from build123d import *

# Parameters (mm, degrees)
SKETCH_W     = 250
SKETCH_H     = 10
SKETCH001_R  = 60
PAD_DEPTH    = 60
SKETCH002_R  = 45
PAD001_DEPTH = 45
SKETCH003_R  = 45
PAD002_DEPTH = 20


with BuildPart() as part:
    # Sketch → Revolution (revolve)
    with BuildSketch(Plane.XY):
        with Locations((125, 35)):
            Rectangle(SKETCH_W, SKETCH_H)
    revolve(axis=Axis((0, 0, 0), (1, 0, 0)))

    # Sketch001 → Pad (new body, symmetric)
    with BuildSketch(Plane.XY):
        Circle(SKETCH001_R)
    extrude(amount=PAD_DEPTH, both=True)

    # Sketch002 → Pad001 (join, symmetric)
    with BuildSketch(Plane.XY):
        with Locations((250, 0)):
            Circle(SKETCH002_R)
    extrude(amount=PAD001_DEPTH, both=True)

    # Sketch003 (on Face6 of Pad001) → Pad002 (join)
    with BuildSketch(Plane(origin=(0, 0, -45), x_dir=(1, 0, 0), z_dir=(0, 0, -1))):
        with Locations((250, 0)):
            Circle(SKETCH003_R)
    extrude(amount=PAD002_DEPTH)


solid = part.part
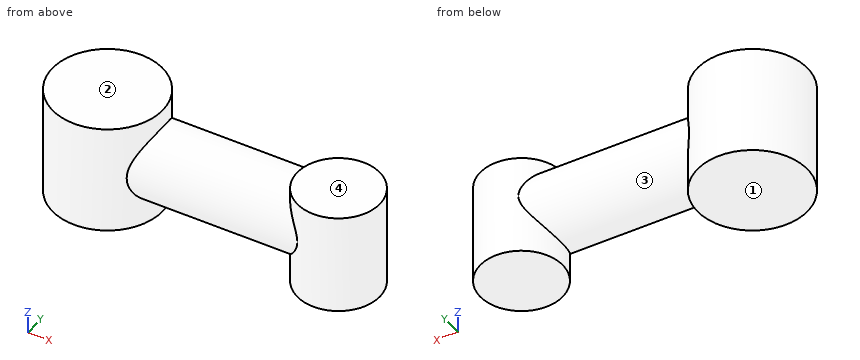
Geometry check sheet. Reference: the model listing, model coordinates, mm. Face numbers are marked on the shaded views. A direction names the side the tool comes from. Coordinates: 2 decimals unless noted, no trailing zeros. Order: outer loops, then holes, each group sorted by start corner. A loop starts at its lowest first (then second) coordinate and runs counter-clockwise, first axis right, second up. Notation, with made-up numbers: (61.5, -0.5) - (106.5, -0.5) arc R14 cw to (106.5, 23.5) - close; hole circle Ø4 at (38.5, 5.5). An arc over 180 degrees is marked (long way). One line per item, written item: value.
(1) Sectioned sample at D-D (z = -52). Enter the section's corners in (x, y).
Data:
outline: circle Ø120 at (0, 0); circle Ø90 at (250, 0)
(2) Access from +Z, -Z, +X, -X, +Y, -Y to the whole of each face (thin tool, end or side, straight path). Record for the marked faces 1 and 2.
Data:
face 1: -Z, -X, +Y, -Y
face 2: +Z, +X, -X, +Y, -Y
(3) Release check for a two-part mould opening along X. For the marked faces 3 and 4 record: +X half, -X half, draft (parallel to the pull), parting line (faces both ways), or undercut.
Data:
face 3: undercut
face 4: draft
(4) Sectioned sample at C-C (x = 136.5). Enter the section's corners in (y, z).
Data:
outline: circle Ø80 at (0, 0); hole circle Ø60 at (0, 0)
(5) Depth check by flat-ended pin: pin 1 Ø8 at (x, y) = (86.5, -5.5) entering from -Z; pin 2 Ø8 at (x, z) = (40.5, 32) entering from -Y; pin 3 Ø1 at (y, z) = (7, -32) entering from -X. Enter the tip coordinate at first touch or a pass-through.
Data:
pin 1: stops at z = -39.97
pin 2: stops at y = -47.62
pin 3: stops at x = -59.65
(6) Thickness scan on probe 1 along Z at (x, y) = (145, 0); probe 2 along Z at (x, y) = (79, -2). Record the ranges inside material, lowest first. Write a range as from..to.
Data:
probe 1: z = -40..-30, 30..40
probe 2: z = -39.95..-29.93, 29.93..39.95
(7) Sectioned sample at B-B (y = 0). Enter the section's corners in (x, z), and give its area (3 significant figures).
Data:
outline: (-60, -60) - (60, -60) - (60, -40) - (205, -40) - (205, -65) - (295, -65) - (295, 45) - (205, 45) - (205, 40) - (60, 40) - (60, 60) - (-60, 60) - close; hole (60, -30) - (205, -30) - (205, 30) - (60, 30) - close
area: 27,200 mm^2
(8) Sectioned sample at A-A (z = 0). Enter the section's corners in (x, y), and give its area (3 significant figures).
Data:
outline: (44.72, -40) - (229.38, -40) arc R45 ccw (long way) to (229.38, 40) - (44.72, 40) arc R60 ccw (long way) to start; hole (51.96, -30) - (216.46, -30) arc R45 cw to (216.46, 30) - (51.96, 30) arc R60 cw to start
area: 21,100 mm^2
